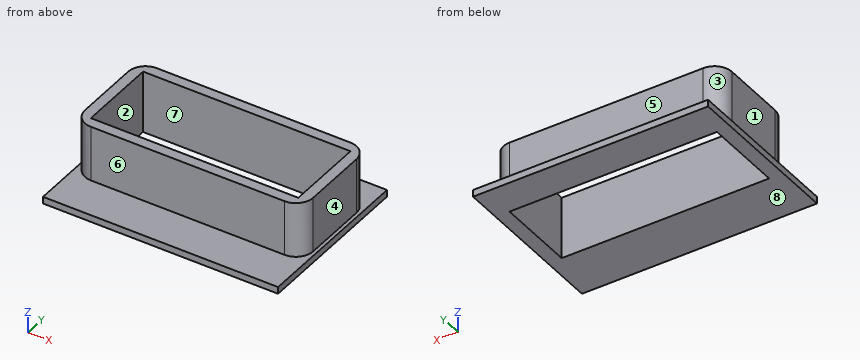
from build123d import *

# Parameters (mm, degrees)
F0_W     = 68
F0_H     = 48
F1_DEPTH = 2
F0_W_2   = 60
F0_H_2   = 23
F2_DEPTH = 18


with BuildPart() as f1:
    # F0 (on Top) → F1 (new body)
    with BuildSketch(Plane.XY):
        with Locations((33, 12)):
            Rectangle(F0_W, F0_H)
        with BuildLine():
            Line((61, 0), (5, 0))
            ThreePointArc((5, 0), (1.464466, 1.464466), (0, 5))
            Line((0, 5), (0, 24))
            ThreePointArc((0, 24), (1.464466, 27.535534), (5, 29))
            Line((5, 29), (61, 29))
            ThreePointArc((61, 29), (64.535534, 27.535534), (66, 24))
            Line((66, 24), (66, 5))
            ThreePointArc((66, 5), (64.535534, 1.464466), (61, 0))
        make_face(mode=Mode.SUBTRACT)
    extrude(amount=F1_DEPTH)

    # F0 (on Top) → F2 (join)
    with BuildSketch(Plane.XY):
        with BuildLine():
            ThreePointArc((0, 5), (1.464466, 1.464466), (5, 0))
            Line((5, 0), (61, 0))
            ThreePointArc((61, 0), (64.535534, 1.464466), (66, 5))
            Line((66, 5), (66, 24))
            ThreePointArc((66, 24), (64.535534, 27.535534), (61, 29))
            Line((61, 29), (5, 29))
            ThreePointArc((5, 29), (1.464466, 27.535534), (0, 24))
            Line((0, 24), (0, 5))
        make_face()
        with Locations((33, 14.5)):
            Rectangle(F0_W_2, F0_H_2, mode=Mode.SUBTRACT)
    extrude(amount=F2_DEPTH)


solid = f1.part
Here's how the part is built. I have some questions about the finished solid (model axes, mm). Face numbers are marked on the shaded views. A direction names the side the tool comes from. Give positions to 0.01 mm unless a question says otherwise; leave off trailing zeros. Write each loop counter-clockwise with the first axis right and the second up, starting at its lowest first coordinate (ties: lowest second). Pieces come first, ordered by that corner, then holes. Notation, with made-up numbers: (8.25, 10.25) -> (47.25, 10.25) arc R27 ccw to (47.25, 28.25) -> close; hole circle Ø5 at (20, 11.5). An arc over 180 degrees is marked (long way). Use one line per item in the form item = value. Start each with the question number.
1. Imagine slicing it at C-C on x = 60. List the corners of the cut face in (y, z) for me.
2. Thinking about a two-plate mould opening in Y: for the marked faces 6, 7 and 8, which applies, +Y half, -Y half, draft (parallel to the pull), parting line (faces both ways), or undercut?
3. Imagine slicing it at D-D on y = -5.5. List the corners of the cut face in (x, z) for me.
4. If I drill on L1, parallel to Y at x = 17.5, z = 9; L2, parallel to X at y = 16, z = 12.75; L3, parallel to X at y = 12, z = 1, over which ranges is the centre line in solid material (lowest first)?
5. Imagine slicing it at A-A on z = 16.5. List the corners of the cut face in (x, y) for me, plus the area to 3 significant figures.
6. On a 3-axis mill with a long thin cutter (end or side, diameter ignored), from which of +Z, -Z, +X, -X, +Y, -Y can I reach the whole of each face in a straight line? I mean the marked faces 1, 2, 3, 4 and 5. Say none if no direction works.
7. Will these pins go through, and if not, where does the flat tip stop? pin 1 Ø8 at (x, z) = (31, 13.5) entering from +Y; pin 2 Ø4 at (x, y) = (23, -5.5) entering from +Z; pin 3 Ø5.5 at (x, z) = (46.5, 5) entering from -Y.
8. Imagine slicing it at B-B on y = 10.5. List the corners of the cut face in (x, z) for me, plus the area to 3 significant figures.
Entries:
q1.outline = (-12, 0) -> (3, 0) -> (3, 18) -> (0, 18) -> (0, 2) -> (-12, 2) -> close; (26, 0) -> (36, 0) -> (36, 2) -> (29, 2) -> (29, 18) -> (26, 18) -> close
q2.face_6 = -Y half
q2.face_7 = undercut
q2.face_8 = draft
q3.outline = (-1, 0) -> (67, 0) -> (67, 2) -> (-1, 2) -> close
q4.L1 = 0 to 3, 26 to 29
q4.L2 = 0 to 3, 63 to 66
q4.L3 = -1 to 3, 63 to 67
q5.outline = (0, 5) arc R5 ccw to (5, 0) -> (61, 0) arc R5 ccw to (66, 5) -> (66, 24) arc R5 ccw to (61, 29) -> (5, 29) arc R5 ccw to (0, 24) -> close; hole (3, 3) -> (63, 3) -> (63, 26) -> (3, 26) -> close
q5.area = 513 mm²
q6.face_1 = +Z, -X, +Y, -Y
q6.face_2 = +Z, -Z
q6.face_3 = +Z, -X, +Y
q6.face_4 = +Z, +X, +Y, -Y
q6.face_5 = +Z, +X, -X, +Y
q7.pin_1 = 29
q7.pin_2 = 2
q7.pin_3 = 0
q8.outline = (-1, 0) -> (3, 0) -> (3, 18) -> (0, 18) -> (0, 2) -> (-1, 2) -> close; (63, 0) -> (67, 0) -> (67, 2) -> (66, 2) -> (66, 18) -> (63, 18) -> close
q8.area = 112 mm²
